Geometry check sheet. Reference: the model listing, model coordinates, mm. A direction names the side the tool comes from. Coordinates: 2 decimals unless noted, no trailing zeros. Write each loop counter-clockwise with the first axis right and the second up, starting at its lowest first coordinate (ties: lowest second). Pieces come first, ordered by that corner, then holes. Notation, with made-up numbers: M 57,75.25 L 71,75.25 A16 cw 71,86.25 Z; hole C 13.5,86 d5. An arc over 180 degrees is marked long. Write each question's results on one line, items separated by ' | '.
```python
from build123d import *

# Parameters (mm, degrees)
CUT_EXTRUDE2_START = -30
CUT_EXTRUDE2_DEPTH = 30
SKETCH5_R          = 3
CUT_EXTRUDE3_DEPTH = 40
CUT_EXTRUDE4_START = -138.75
SKETCH6_R          = 12
SKETCH6_R_2        = 8
CUT_EXTRUDE4_DEPTH = 138.75
CUT_EXTRUDE5_DEPTH = 15
FILLET1_R          = 1
SKETCH8_R          = 2.5
CUT_EXTRUDE6_DEPTH = 1


with BuildPart() as part:
    # Sketch2 → Revolve2 (revolve)
    with BuildSketch(Plane(origin=(0, 0, 0), x_dir=(1, 0, 0), z_dir=(0, 1, 0)), mode=Mode.PRIVATE) as revolve2_sk:
        Polygon((0, -277.5), (8, -277.5), (8, -262.5), (12, -262.5), (12, 262.5), (8, 262.5), (8, 277.5), (0, 277.5), align=None)
    revolve(revolve2_sk.sketch.rotate(Axis((0, 0, -364.100348117), (0, 0, 1)), 180), axis=Axis((0, 0, -364.100348117), (0, 0, 1)))

    # Sketch4 → Cut-Extrude2 (cut)
    with BuildSketch(Plane.XY.offset(277.5).offset(CUT_EXTRUDE2_START)):
        with BuildLine():
            Line((-6.488318348, 1.39), (-7.878318348, 1.39))
            ThreePointArc((-7.878318348, 1.39), (-8, 0), (-7.878318348, -1.39))
            Line((-7.878318348, -1.39), (-6.488318348, -1.39))
            Line((-6.488318348, -1.39), (-6.488318348, 1.39))
        make_face()
    extrude(amount=CUT_EXTRUDE2_DEPTH, mode=Mode.SUBTRACT)

    # Sketch5 → Cut-Extrude3 (cut)
    with BuildSketch(Plane.XY.offset(277.5)):
        Circle(SKETCH5_R)
    extrude(amount=-CUT_EXTRUDE3_DEPTH, mode=Mode.SUBTRACT)

    # Sketch6 → Cut-Extrude4 (cut)
    with BuildSketch(Plane.XY.offset(262.5).offset(CUT_EXTRUDE4_START)):
        with Locations(Location((0, 0, 0), (0, 0, 180))):
            Circle(SKETCH6_R)
        with Locations(Location((0, 0, 0), (0, 0, 180))):
            Circle(SKETCH6_R_2, mode=Mode.SUBTRACT)
    extrude(amount=CUT_EXTRUDE4_DEPTH, mode=Mode.SUBTRACT)

    # Sketch7 → Cut-Extrude5 (cut)
    with BuildSketch(Plane(origin=(0, 0, -277.5), x_dir=(-1, 0, 0), z_dir=(0, 0, -1))):
        with BuildLine():
            Line((-4, 6.92820323), (-4, -6.92820323))
            ThreePointArc((-4, -6.92820323), (-8, 0), (-4, 6.92820323))
        make_face()
        with BuildLine():
            Line((4, -6.92820323), (4, 6.92820323))
            ThreePointArc((4, 6.92820323), (8, 0), (4, -6.92820323))
        make_face()
    extrude(amount=-CUT_EXTRUDE5_DEPTH, mode=Mode.SUBTRACT)

    # Fillet1
    fillet1_edges = [part.edges().sort_by_distance(p)[0] for p in [
        (4, 6.92820323, -270),
        (4, -6.92820323, -270),
        (-4, -6.92820323, -270),
        (-4, 6.92820323, -270),
    ]]
    fillet(fillet1_edges, radius=FILLET1_R)

    # Sketch8 → Cut-Extrude6 (cut)
    with BuildSketch(Plane(origin=(4, 0, 0), x_dir=(0, 0, -1), z_dir=(1, 0, 0))):
        with Locations((270, 0)):
            Circle(SKETCH8_R)
    extrude(amount=-CUT_EXTRUDE6_DEPTH, mode=Mode.SUBTRACT)


solid = part.part
```
Q1. Access from +Z, -Z, +X, -X, +Y, -Y to the whole of each face (thin tool, end or side, straight path). Record for faces 1 (the flat face through (-4, 0, -270)), 2 (the flat face through (-0.1, 3.4, 277.5)), 3 (the cylindrical face through (-11.446, -3.604, -72.079)), 4 (the flat face through (4, 3, -270)), 5 (the flat face through (-8, 2, 123.75)).
Geometry check:
face 1: -Z, -X, +Y, -Y | face 2: +Z, +X, -X, +Y, -Y | face 3: +Z, -Z | face 4: -Z, +X, +Y, -Y | face 5: +Z
Q2. Sectioned sample at B-B on z = 200. Record the cut outline in (x, y).
Geometry check:
outline: C 0,0 d16
Q3. Scan lines: probe 1 along Y at (x, z) = (0, 263); probe 2 along Y at (x, z) = (3.4, -270); probe 3 along Z at (x, y) = (6, 0.75). Record each from-to range of solid material in increasing order.
Geometry check:
probe 1: y = -8 to -3, 3 to 8 | probe 2: y = -7.24 to -2.5, 2.5 to 7.24 | probe 3: z = -262.5 to 277.5
Q4. Depth check by flat-ended pin: P1, Ø6, axis at y = 0, z = -270, coming from the -X side; P2, Ø5, axis at x = 4.5, z = 0, coming from the +Y side; P3, Ø5, axis at x = -0.5, z = 133.5, coming from the +Y side. Enter the tip coordinate at first touch or a pass-through.
Geometry check:
P1: stops at x = -4 | P2: stops at y = 11.83 | P3: stops at y = 8
Q5. Sectioned sample at A-A on z = -234. Record the cut outline in (x, y), and give its area (3 significant figures).
Geometry check:
outline: C 0,0 d24 | area: 452 mm2
